Here's the drawing with two shaded views (mm, measured from the low corner). I have some questions. A direction names the side the tool comes from. Give positions to 0.01 mm unless a question says otherwise; leave off trailing zeros. Write each loop counter-clockwise with the first axis right and the second up, starting at its lowest first coordinate (ties: lowest second). Pieces come first, ordered by that corner, then holes.
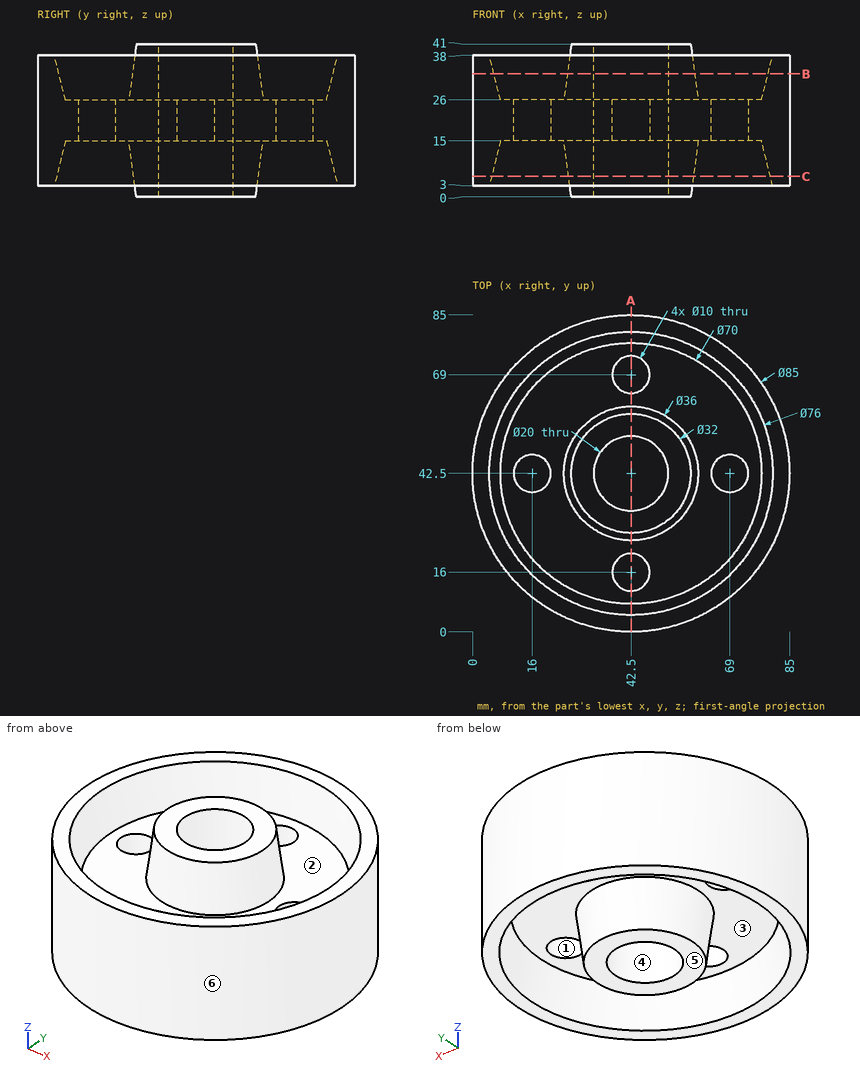
1) For pin 1 Ø8 at (y, z) = (16.5, 8.5) entering from +X; pin 2 Ø1 at (y, z) = (71, 32) entering from -X; pin 3 Ø8 at (x, y) = (42.5, 16) entering from -Z; pin 4 Ø10 at (y, z) = (17, 12.5) entering from -X, each with a flat end and sliding along its axis, tell me the tip position at first contact or that it passes through.
Values follow:
pin 1: stops at x = 78.86
pin 2: stops at x = 10.53
pin 3: passes through
pin 4: stops at x = 5.27
2) Please list where these lines run through material, in increasing order: L1, parallel to Y at x = 42.5, z = 19; L2, parallel to X at y = 42, z = 18; L3, parallel to Y at x = 48.5, z = 12.
Values follow:
L1: y = 0 to 11, 21 to 32.5, 52.5 to 64, 74 to 85
L2: x = 0 to 11.03, 20.97 to 32.51, 52.49 to 64.03, 73.97 to 85
L3: y = 0.43 to 7.26, 25.95 to 34.5, 50.5 to 59.05, 77.74 to 84.57
3) For the marked faces 1, 2 and 3, which set-ups out of +Z, -Z, +X, -X, +Y, -Y let a thin tool reach every point of the face, with its end or its side?
Values follow:
face 1: +Z, -Z
face 2: +Z
face 3: -Z
4) If we mould it in two halves opening along Y, with no side actions, what happens to the marked faces 4, 5 and 6? For each: +Y half, -Y half, draft (parallel to the pull), parting line (faces both ways), or undercut.
Values follow:
face 4: undercut
face 5: draft
face 6: parting line
5) Suppose I cut it at B-B on z = 33. Write out the boundary of the cut face in (x, y).
Values follow:
outline: circle Ø85 at (42.5, 42.5); circle Ø34.13 at (42.5, 42.5); hole circle Ø73.5 at (42.5, 42.5); hole circle Ø20 at (42.5, 42.5)
6) Suppose I cut it at A-A on x = 42.5. State how many separate pieces and enclosed holes the cut face has, plus the area to 3 significant figures.
Values follow:
separate pieces: 4
enclosed holes: 0
area: 1,200 mm2
7) Suppose I cut it at C-C on z = 5.5. Write out the boundary of the cut face in (x, y) (3 decimals), plus the area to 3 significant figures.
Values follow:
outline: circle Ø85 at (42.5, 42.5); circle Ø33.467 at (42.5, 42.5); hole circle Ø74.75 at (42.5, 42.5); hole circle Ø20 at (42.5, 42.5)
area: 1,850 mm2
